Autodesk Inventor part; units mm, degrees
ref_plane "YZ Plane" through (0, 0, 0) normal (1, 0, 0) x (0, 1, 0)
ref_plane "XZ Plane" through (0, 0, 0) normal (0, 1, 0) x (-1, 0, 0)
ref_plane "XY Plane" through (0, 0, 0) normal (0, 0, 1) x (1, 0, 0)
sketch "Sketch1" plane through (0, 0, 0) normal (0, 0, 1) x (1, 0, 0)
  circle A0 centre (0, 0) radius 77
  dimension "d0" = 154
extrude "Extrusion1" add sketch "Sketch1" along normal blind 2
sketch "Sketch2" plane through (0, 0, 2) normal (0, 0, 1) x (1, 0, 0)
  circle A0 centre (0, 0) radius 77
  circle A1 centre (0, 0) radius 75
  dimension "d4" = 150
extrude "Extrusion2" add sketch "Sketch2" along normal blind 8 contours A1
sketch "Sketch3" plane through (0, 0, 10) normal (0, 0, 1) x (1, 0, 0)
  circle A0 centre (0, 0) radius 77
extrude "Extrusion3" add sketch "Sketch3" along normal blind 2
sketch "Sketch4" plane through (0, 0, 0) normal (0, 0, -1) x (-1, 0, 0)
  circle A0 centre (0, 0) radius 77
  line L0 (75.9786, 12.5) -> (0, 12.5)
  arc A1 (0, 12.5) -> (0, -12.5) centre (0, 0) ccw
  line L1 (0, -12.5) -> (75.9786, -12.5)
  dimension "d10" = 12.5
properties part number "pulley template"
Could you check a few things on this model? Use its own coordinates, in mm. A direction names the side the tool comes from. Give positions to 0.01 mm unless a question says otherwise; leave off trailing zeros. Order: outer loops, then holes, each group sorted by start corner. A loop starts at its lowest first (then second) coordinate and runs counter-clockwise, first axis right, second up.
Q1. If I drill on line 1 along X through (y, z) = (35, 7); line 2 along Y through (x, z) = (-13, 4.25); line 3 along X through (y, z) = (-16, 3.25), over which ranges is the centre line in solid material (lowest first)?
Q2. I'm going to push flat-ended pins straight in: P1, Ø1, axis at x = -59.5, z = 2, coming from the -Y side; P2, Ø4, axis at x = 50, z = 5, coming from the -Y side; P3, Ø6, axis at y = 55, z = 6, coming from the +X side. Where does each tip first touch, or does it pass through?
Q3. We'd pull the mould along Z, two halves only. Please class faces 1 (the flat face through (17, -74, 2)), 2 (the flat face through (-1, 1, 12)), 3 (the cylindrical face through (-61.105, 46.853, 10.986)), 4 (the flat face through (17, -74, 10)): +Z half, -Z half, draft (parallel to the pull), parting line (faces both ways), or undercut.
Q4. For faces 5 (the cylindrical face through (-9.764, -74.362, 5.944)), 6 (the flat face through (-1, 1, 0)), which set-ups out of +Z, -Z, +X, -X, +Y, -Y let a thin tool reach every point of the face, with its end or its side?
Q5. Suppose I cut it at C-C, the plane z = 4. Write out the boundary of the cut face in (x, y).
Q6. Suppose I cut it at A-A, the plane x = 0. Write out the boundary of the cut face in (y, z), and give its area (3 significant figures).
Solution:
1. line 1: x = -66.33 to 66.33
1. line 2: y = -73.86 to 73.86
1. line 3: x = -73.27 to 73.27
2. P1: stops at y = -49.48
2. P2: stops at y = -57.63
2. P3: stops at x = 54.05
3. face 1: undercut
3. face 2: +Z half
3. face 3: draft
3. face 4: undercut
4. face 5: none
4. face 6: -Z, +X, -X, +Y, -Y
5. outline: circle Ø150 at (0, 0)
6. outline: (-77, 0) - (77, 0) - (77, 2) - (75, 2) - (75, 10) - (77, 10) - (77, 12) - (-77, 12) - (-77, 10) - (-75, 10) - (-75, 2) - (-77, 2) - close
6. area: 1,820 mm2
